```python
from build123d import *

# Parameters (mm, degrees)
BOSS_EXTRUDE1_DEPTH     = 35
CUT_EXTRUDE1_DEPTH      = 55.01490535
CUT_EXTRUDE1_DEPTH_BACK = 55.01490535
SKETCH4_R               = 3
CHAMFER1_SIZE           = 25
FILLET1_R               = 20
FILLET2_R               = 5.5
FILLET3_R               = 1
CUT_EXTRUDE2_DEPTH      = 59.587029281
CUT_EXTRUDE2_DEPTH_BACK = 59.587029281
FILLET4_R               = 4


with BuildPart() as part:
    # Sketch3 → Boss-Extrude1 (new body)
    with BuildSketch(Plane(origin=(0, 0, 0), x_dir=(1, 0, 0), z_dir=(0, 1, 0))):
        Polygon((39, -13.1), (39, -9.1), (4, -9.1), (4, 9.1), (39, 9.1), (39, 13.1), (0, 13.1), (0, -13.1), align=None)
    extrude(amount=BOSS_EXTRUDE1_DEPTH)

    # Sketch4 → Cut-Extrude1 (cut, two sides: drawn at the far end of the back side and taken through both)
    with BuildSketch(Plane.XY.offset(-CUT_EXTRUDE1_DEPTH_BACK)):
        with Locations((31, 25)):
            Circle(SKETCH4_R)
    extrude(amount=CUT_EXTRUDE1_DEPTH + CUT_EXTRUDE1_DEPTH_BACK, mode=Mode.SUBTRACT)

    # Chamfer1
    # the kernel refuses this chamfer: 25 mm, written as the material it takes off along each edge
    with BuildSketch(Plane(origin=(0, 35, -77.392074699), x_dir=(0.9996219169112966, 0.027495876610586317, 0), z_dir=(0, 0, 1))) as chamfer1_piece_1:
        Polygon((CHAMFER1_SIZE * 0.999621916911, -CHAMFER1_SIZE * 0.0274958766106), (-CHAMFER1_SIZE * 0.0274958766106, -CHAMFER1_SIZE * 0.999621916911), (0, 0), align=None)
    extrude(amount=154.784149398, mode=Mode.SUBTRACT)

    # Fillet1
    # the kernel refuses this fillet: 20 mm, written as the material it takes off along each edge
    with BuildSketch(Plane(origin=(0, 10, -33.810678119), x_dir=(0.7071067811862652, 0.7071067811868299, 0), z_dir=(0, 0, 1))) as fillet1_piece_1:
        with BuildLine():
            CenterArc((FILLET1_R * 0.414213562373, -FILLET1_R), FILLET1_R, 90, 45)
            Line((-FILLET1_R * 0.292893218813, -FILLET1_R * 0.292893218813), (0, 0))
            Line((0, 0), (FILLET1_R * 0.414213562373, 0))
        make_face()
    extrude(amount=67.621356237, mode=Mode.SUBTRACT)
    with BuildSketch(Plane(origin=(25, 35, -33.810678119), x_dir=(-0.7071067811862648, -0.7071067811868303, 0), z_dir=(0, 0, 1))) as fillet1_piece_2:
        with BuildLine():
            CenterArc((FILLET1_R * 0.414213562373, FILLET1_R), FILLET1_R, 225, 45)
            Line((-FILLET1_R * 0.292893218814, FILLET1_R * 0.292893218814), (0, 0))
            Line((0, 0), (FILLET1_R * 0.414213562373, 0))
        make_face()
    extrude(amount=45.421356237, mode=Mode.SUBTRACT)
    with BuildSketch(Plane(origin=(25, 35, -11.610678119), x_dir=(1, 0, 0), z_dir=(0, 0, 1))) as fillet1_piece_3:
        with BuildLine():
            CenterArc((FILLET1_R * 0.414213562373, -FILLET1_R), FILLET1_R, 90, 45)
            Line((-FILLET1_R * 0.292893218814, -FILLET1_R * 0.292893218814), (0, 0))
            Line((0, 0), (FILLET1_R * 0.414213562373, 0))
        make_face()
    extrude(amount=45.421356237, mode=Mode.SUBTRACT)

    # Fillet2
    fillet2_edges = [part.edges().sort_by_distance(p)[0] for p in [
        (39, 35, -11.1),
        (39, 35, 11.1),
    ]]
    fillet(fillet2_edges, radius=FILLET2_R)

    # Fillet3
    fillet3_edges = [part.edges().sort_by_distance(p)[0] for p in [
        (4, 13.715728753, 0),
    ]]
    fillet(fillet3_edges, radius=FILLET3_R)

    # Sketch5 → Cut-Extrude2 (cut, two sides: drawn at the far end of the back side and taken through both)
    with BuildSketch(Plane.XY.offset(13.1).offset(-CUT_EXTRUDE2_DEPTH_BACK)):
        with BuildLine():
            Line((4, 4), (35, 4))
            Line((35, 4), (35, 18))
            ThreePointArc((35, 18), (16.600505063, 17.420310217), (4, 4))
        make_face()
    extrude(amount=CUT_EXTRUDE2_DEPTH + CUT_EXTRUDE2_DEPTH_BACK, mode=Mode.SUBTRACT)

    # Fillet4
    fillet4_edges = [part.edges().sort_by_distance(p)[0] for p in [
        (4, 4, 11.1),
        (4, 4, -11.1),
        (35, 18, 11.1),
        (35, 4, 11.1),
    ]]
    fillet(fillet4_edges, radius=FILLET4_R)


solid = part.part
```
Check sheet for the modelled part. Datum: model origin and axes. Units: mm. A direction names the side the tool comes from. Give positions to 0.01 mm unless a question says otherwise; leave off trailing zeros. Order: outer loops, then holes, each group sorted by start corner. A loop starts at its lowest first (then second) coordinate and runs counter-clockwise, first axis right, second up. Notation, with made-up numbers: M 20,86.5 L 42,86.5 A24 ccw 42,122.5 Z; hole C 26.5,66.5 d2. An arc over 180 degrees is marked long. Answer in a Markdown table with one row per item. Add a question column.
Q1. Access from +Z, -Z, +X, -X, +Y, -Y to the whole of each face (thin tool, end or side, straight path). Record for faces 1 (the flat face through (39, 15, -11)), 2 (the flat face through (35, 11, 11)), 3 (the cylindrical face through (3.21, 11.18, -0.13)).
Q2. Sectioned sample at C-C, the plane y = 21. Record the boundary of the cut face in (x, z), and give its area (3 significant figures).
Q3. Thickness scan on L1, parallel to Z at x = 11.5, y = 16.5; L2, parallel to Y at x = 31, z = 10; L3, parallel to Y at x = 18, z = 9.5. Record the ranges inside material, lowest first.
Q4. Sectioned sample at A-A, the plane z = 11. Record the boundary of the cut face in (x, y).
Q5. Release check for a two-part mould opening along X. For faces 4 (the flat face through (4, 5, 0)), 5 (the flat face through (21, 4, 11)), 6 (the flat face through (24, 21, -13.1)) record: released by +X, released by -X, zero draft, split by the parting line, or undercut.
Q6. Sectioned sample at B-B, the plane y = 25. Record the boundary of the cut face in (x, z).
Q7. Gauge pin test, flat ends, axial feed: pin 1 Ø4.5 at (x, z) = (18, 12) entering from +Y; pin 2 Ø11 at (y, z) = (3.5, 2.5) entering from +X; pin 3 Ø2 at (y, z) = (13, -12) entering from -X. Record the tip position at first contact, or that the pin passes through.
Q8. Sectioned sample at D-D, the plane x = 25. Record the boundary of the cut face in (y, z), and give its area (3 significant figures).
Verdict:
| question | item | result |
|---|---|---|
| 1 | face 1 | +Z, -Z, +X, +Y, -Y |
| 1 | face 2 | +Z, -Z |
| 1 | face 3 | +Y |
| 2 | outline | M 11,-13.1 L 39,-13.1 L 39,-9.1 L 11,-9.1 Z; M 11,9.1 L 39,9.1 L 39,13.1 L 11,13.1 Z |
| 2 | area | 224 mm² |
| 3 | L1 | -13.1 to -9.1, 9.1 to 13.1 |
| 3 | L2 | 0 to 4, 19.13 to 22, 28 to 34.87 |
| 3 | L3 | 0 to 4, 18 to 28 |
| 4 | outline | M 0,0 L 39,0 L 39,29.5 A5.5 ccw 33.5,35 L 33.28,35 A20 ccw 19.14,29.14 L 5.86,15.86 A20 ccw 0,1.72 Z; hole M 7.69,10.49 A4 ccw 10.82,4 L 31,4 A4 ccw 35,8 L 35,15.04 A4 ccw 31.9,18.94 A24.05 ccw Z; hole C 31,25 d6 |
| 5 | face 4 | released by +X |
| 5 | face 5 | undercut |
| 5 | face 6 | zero draft |
| 6 | outline | M 15,-13.1 L 28,-13.1 L 28,-9.1 L 15,-9.1 Z; M 15,9.1 L 28,9.1 L 28,13.1 L 15,13.1 Z; M 34,-13.1 L 39,-13.1 L 39,-9.1 L 34,-9.1 Z; M 34,9.1 L 39,9.1 L 39,13.1 L 34,13.1 Z |
| 7 | pin 1 | y = 30.17 |
| 7 | pin 2 | x = 4 |
| 7 | pin 3 | x = 2.85 |
| 8 | outline | M 0,-13.1 L 4,-13.1 L 4,-9.1 L 0,-9.1 Z; M 0,9.1 L 4,9.1 L 4,13.1 L 0,13.1 Z; M 19.51,-13.1 L 33.2,-13.1 L 33.2,-9.1 L 19.51,-9.1 Z; M 19.51,9.1 L 33.2,9.1 L 33.2,13.1 L 19.51,13.1 Z |
| 8 | area | 142 mm² |
